from build123d import *

# Parameters (mm, degrees)
F0_R      = 13.525
F0_R_2    = 6.35
F1_DEPTH  = 23.8
F2_R      = 13.525
F2_R_2    = 7.95
F3_DEPTH  = 2
F4_R      = 13.525
F4_R_2    = 12.75
F5_DEPTH  = 1.2
F6_R      = 1.1608870099
F6_R_2    = 13.525
F6_R_3    = 6.35
F7_DEPTH  = 4.75
F8_R      = 12.75
F8_R_2    = 6.35
F9_DEPTH  = 1.2
F10_R     = 7.925
F10_R_2   = 6.35
F11_DEPTH = 2.5
F13_R     = 13.525
F13_R_2   = 12.75
F14_DEPTH = 1.2


with BuildPart() as f1:
    # F0 (on Top) → F1 (new body)
    with BuildSketch(Plane.XY):
        Circle(F0_R)
        Circle(F0_R_2, mode=Mode.SUBTRACT)
    extrude(amount=F1_DEPTH)

    # F2 (on face) → F3 (cut)
    with BuildSketch(Plane.XY.offset(23.8)):
        Circle(F2_R)
        Circle(F2_R_2, mode=Mode.SUBTRACT)
    extrude(amount=-F3_DEPTH, mode=Mode.SUBTRACT)

    # F4 (on face) → F5 (cut)
    with BuildSketch(Plane.XY.offset(21.8)):
        Circle(F4_R)
        Circle(F4_R_2, mode=Mode.SUBTRACT)
    extrude(amount=-F5_DEPTH, mode=Mode.SUBTRACT)

    # F6 (on face) → F7 (join)
    with BuildSketch(Plane(origin=(0, 0, 0), x_dir=(1, 0, 0), z_dir=(0, 0, -1))):
        with BuildLine():
            Line((21.1923624897, -5.9062485645), (5.4812199469, 21.3062485645))
            ThreePointArc((5.4812199469, 21.3062485645), (0, 22), (-5.4812199469, 21.3062485645))
            Line((-5.4812199469, 21.3062485645), (-21.1923624897, -5.9062485645))
            ThreePointArc((-21.1923624897, -5.9062485645), (-19.0525588833, -11), (-15.7111425428, -15.4))
            Line((-15.7111425428, -15.4), (15.7111425428, -15.4))
            ThreePointArc((15.7111425428, -15.4), (19.0525588833, -11), (21.1923624897, -5.9062485645))
        make_face()
        with Locations((-14.2461178923, -8.225)):
            Circle(F6_R, mode=Mode.SUBTRACT)
        with Locations((14.2461178923, -8.225)):
            Circle(F6_R, mode=Mode.SUBTRACT)
        Circle(F6_R_2, mode=Mode.SUBTRACT)
        with Locations((0, 16.45)):
            Circle(F6_R, mode=Mode.SUBTRACT)
        Circle(F6_R_2)
        Circle(F6_R_3, mode=Mode.SUBTRACT)
    extrude(amount=F7_DEPTH)

    # F8 (on face) → F9 (cut)
    with BuildSketch(Plane(origin=(0, 0, -4.75), x_dir=(1, 0, 0), z_dir=(0, 0, -1))):
        Circle(F8_R)
        Circle(F8_R_2, mode=Mode.SUBTRACT)
    extrude(amount=-F9_DEPTH, mode=Mode.SUBTRACT)

    # F10 (on face) → F11 (cut)
    with BuildSketch(Plane(origin=(0, 0, -3.55), x_dir=(1, 0, 0), z_dir=(0, 0, -1))):
        Circle(F10_R)
        Circle(F10_R_2, mode=Mode.SUBTRACT)
    extrude(amount=-F11_DEPTH, mode=Mode.SUBTRACT)

    # F13 (on offset) → F14 (cut)
    with BuildSketch(Plane.XY.offset(17.8)):
        Circle(F13_R)
        Circle(F13_R_2, mode=Mode.SUBTRACT)
    extrude(amount=-F14_DEPTH, mode=Mode.SUBTRACT)


solid = f1.part
Read the model definition and answer for the solid it produces. Units are mm, in the model's axes. A direction names the side the tool comes from. Coordinates: 2 decimals unless noted, no trailing zeros. Write each loop counter-clockwise with the first axis right and the second up, starting at its lowest first coordinate (ties: lowest second). Pieces come first, ordered by that corner, then holes. Notation, with made-up numbers: M 5.25,25.5 L 29.25,25.5 A24 cw 29.25,63.5 Z; hole C 26.25,-33.75 d1. An arc over 180 degrees is marked long. Use a Markdown table: item, result.
Q1. Straight lines are drawn through the part: L1, parallel to Y at x = 0, z = -3.85; L2, parallel to Y at x = 0, z = -1.95 (3 decimals); L3, parallel to Z at x = 4, y = -5. For each, find the intervals that lie inside material, in ascending order. Write a range as [from, to].
Answer block:
| item | result |
|---|---|
| L1 | y = [-22, -17.61], [-15.29, -12.75], [12.75, 15.4] |
| L2 | y = [-22, -17.611], [-15.289, -7.925], [7.925, 15.4] |
| L3 | z = [-1.05, 23.8] |
Q2. Each of these flat-tipped pins is pushed along its axis until it touches: pin 1 Ø8 at (x, y) = (-1, -2.5) entering from -Z; pin 2 Ø18 at (x, y) = (0, 0) entering from -Z; pin 3 Ø4 at (y, z) = (-16.5, 2.5) entering from +X; pin 4 Ø2.5 at (x, y) = (0, -16.45) entering from +Z. Where does it stop, or does it pass through?
Answer block:
| item | result |
|---|---|
| pin 1 | stops at z = -1.05 |
| pin 2 | stops at z = -3.55 |
| pin 3 | passes through |
| pin 4 | stops at z = 0 |
Q3. The part is cut by section B-B, the plane x = 0. Give the number of separate pieces and of enclosed holes in the cut face, then the cut area to 3 significant figures.
Answer block:
| item | result |
|---|---|
| separate pieces | 3 |
| enclosed holes | 0 |
| area | 399 mm2 |
Q4. The part is cut by section A-A, the plane y = -17. Write down the section's boundary in (x, z).
Answer block:
| item | result |
|---|---|
| outline | M -7.97,-4.75 L -1.02,-4.75 L -1.02,0 L -7.97,0 Z; M 1.02,-4.75 L 7.97,-4.75 L 7.97,0 L 1.02,0 Z |
Q5. The part is cut by section C-C, the plane z = 19.25. Write down the section's boundary in (x, y) (3 decimals), then the cut area to 3 significant figures.
Answer block:
| item | result |
|---|---|
| outline | C 0,0 d27.05; hole C 0,0 d12.7 |
| area | 448 mm2 |
Q6. Which of the six approach directions +Z, -Z, +X, -X, +Y, -Y give full straight-line access (tool end or side, diameter ignored) to faces 1 (the face through (-8.1, 10.1, 20.6)), 2 (the face through (7.56, -2.38, -2.32)), 3 (the face through (-0.15, -17.6, -2.34)), 4 (the face through (-19.091, 10.933, -2.342)), 5 (the face through (-2.764, -12.447, 17.208))?
Answer block:
| item | result |
|---|---|
| face 1 | +Z |
| face 2 | -Z |
| face 3 | +Z, -Z |
| face 4 | +Z, -Z, -X, +Y |
| face 5 | none |
Q7. Determine the mould class of faces 6 (the face through (-1.38, 6.2, 11.55)), 7 (the face through (-8.1, 10.1, 16.6)), 8 (the face through (-13, -5, 0)) for opening direction Z: released by +Z, released by -Z, zero draft, split by the parting line, or undercut.
Answer block:
| item | result |
|---|---|
| face 6 | zero draft |
| face 7 | undercut |
| face 8 | released by +Z |
Q8. The part is cut by section D-D, the plane z = -2.5. Write down the section's boundary in (x, y) (3 decimals), then the cut area to 3 significant figures.
Answer block:
| item | result |
|---|---|
| outline | M -21.192,5.906 L -5.481,-21.306 A22 ccw 5.481,-21.306 L 21.192,5.906 A22 ccw 15.711,15.4 L -15.711,15.4 A22 ccw Z; hole C -14.246,8.225 d2.322; hole C 0,0 d15.85; hole C 0,-16.45 d2.322; hole C 14.246,8.225 d2.322 |
| area | 881 mm2 |
